Read the model definition and answer for the solid it produces. Units are mm, in the model's axes. A direction names the side the tool comes from. Give positions to 0.01 mm unless a question says otherwise; leave off trailing zeros. Loops run counter-clockwise (first coordinate to the right, second up) from the corner with the lowest first, then second, coordinate; pieces in that order, holes last.
(1) Find section B-B, the plane x = 16. Write down the section's boundary in (y, z).
(2) Which of the six approach directions +Z, -Z, +X, -X, +Y, -Y give full straight-line access (tool end or side, diameter ignored) to faces 1 (the face through (5, -140, 16)), 2 (the face through (10.5, -85, 43)), 3 (the face through (19, -87, 53))?
(3) Find section C-C, the plane y = -72. Write down the section's boundary in (x, z), then the cut area to 3 significant figures.
(4) Straight lines are drawn through the part: probe 1 along Y at (x, z) = (4, 33.5); probe 2 along Y at (x, z) = (21.5, 55); probe 3 along X at (y, z) = (-47.5, 45.5). For each, find the intervals that lie inside material, in ascending order.
(5) Each of these flat-tipped pins is pushed along its axis until it touches: P1, Ø12, axis at x = 15.5, y = -73.5, coming from the -Z side; P2, Ø8, axis at x = 21.5, z = 39, coming from the +Y side; P3, Ø3, axis at x = 19.5, y = -57.5, coming from the -Z side. Where does it stop, or does it pass through?
(6) Find section D-D, the plane z = 58.5. Write down the section's boundary in (x, y), then the cut area to 3 significant figures.
(7) Determine the mould class of faces 4 (the face through (5, -32, 17)), 5 (the face through (5, -87, 38)), 6 (the face through (24, -85, 45.75)), 7 (the face through (10, 0, 39)) for opening direction Y: pulls with the +Y half, pulls with the -Y half, needs draft (parallel to the pull), parting line crosses it, or undercut.
(8) Find section A-A, the plane z = 8. Write down the section's boundary in (x, y), then the cut area to 3 significant figures.
```python
from build123d import *

# Parameters (mm, degrees)
F1_DEPTH = 172.25
F3_DEPTH = 50
F5_DEPTH = 25


with BuildPart() as f1:
    # F0 (on Front) → F1 (new body)
    with BuildSketch(Plane.XZ):
        Polygon((0, 63), (0, 0), (10.5, 0), (10.5, 45.75), (37, 45.75), (37, 63), align=None)
    extrude(amount=F1_DEPTH)

    # F2 (on face) → F3 (cut)
    with BuildSketch(Plane.YZ.offset(37)):
        with BuildLine():
            Line((-20.25, 63), (-152, 63))
            Line((-152, 63), (-152, 55))
            ThreePointArc((-152, 55), (-151.414214, 53.585786), (-150, 53))
            Line((-150, 53), (-22.25, 53))
            ThreePointArc((-22.25, 53), (-20.835786, 53.585786), (-20.25, 55))
            Line((-20.25, 55), (-20.25, 63))
        make_face()
    extrude(amount=-F3_DEPTH, mode=Mode.SUBTRACT)

    # F4 (on face) → F5 (cut)
    with BuildSketch(Plane(origin=(0, 0, 0), x_dir=(0, -1, 0), z_dir=(-1, 0, 0))):
        with BuildLine():
            Line((32, 33), (32, 0))
            Line((32, 0), (140, 0))
            Line((140, 0), (140, 33))
            ThreePointArc((140, 33), (138.535534, 36.535534), (135, 38))
            Line((135, 38), (37, 38))
            ThreePointArc((37, 38), (33.464466, 36.535534), (32, 33))
        make_face()
    extrude(amount=-F5_DEPTH, mode=Mode.SUBTRACT)


solid = f1.part
```
Entries:
1. outline: (-172.25, 45.75) - (0, 45.75) - (0, 63) - (-20.25, 63) - (-20.25, 55) arc R2 cw to (-22.25, 53) - (-150, 53) arc R2 cw to (-152, 55) - (-152, 63) - (-172.25, 63) - close
2. face 1: -Z, +X, -X
2. face 2: -Z, +X, +Y, -Y
2. face 3: +Z, +X, -X
3. outline: (0, 38) - (10.5, 38) - (10.5, 45.75) - (37, 45.75) - (37, 53) - (0, 53) - close
3. area: 350 mm2
4. probe 1: y = -172.25 to -139.97, -32.03 to 0
4. probe 2: y = -172.25 to -152, -20.25 to 0
4. probe 3: x = 0 to 10.5
5. P1: stops at z = 38
5. P2: passes through
5. P3: stops at z = 45.75
6. outline: (0, -172.25) - (37, -172.25) - (37, -152) - (0, -152) - close; (0, -20.25) - (37, -20.25) - (37, 0) - (0, 0) - close
6. area: 1,500 mm2
7. face 4: undercut
7. face 5: undercut
7. face 6: needs draft
7. face 7: pulls with the +Y half
8. outline: (0, -172.25) - (10.5, -172.25) - (10.5, -140) - (0, -140) - close; (0, -32) - (10.5, -32) - (10.5, 0) - (0, 0) - close
8. area: 675 mm2
